Design review of the part built by this model. Coordinates are the model's own, in mm. Coordinates: 2 decimals unless noted, no trailing zeros. Loops run counter-clockwise (first coordinate to the right, second up) from the corner with the lowest first, then second, coordinate; pieces in that order, holes last. Notation, with made-up numbers: M 33,-5 L 80,-5 A9 cw 80,5 Z; hole C 77.25,27.5 d8. An arc over 180 degrees is marked long. Write item = value, one per line. Start each with the question number.
from build123d import *

# Parameters (mm, degrees)
SKETCH1_W           = 38.1
SKETCH1_H           = 28.575
SKETCH1_R           = 3.175
BOSS_EXTRUDE1_DEPTH = 3.175
SKETCH2_R           = 1.8415
CUT_EXTRUDE1_DEPTH  = 25.023234196


with BuildPart() as part:
    # Sketch1 → Boss-Extrude1 (new body)
    with BuildSketch(Plane(origin=(0, 0, 0), x_dir=(1, 0, 0), z_dir=(0, 1, 0))):
        Rectangle(SKETCH1_W, SKETCH1_H)
        with Locations(Location((-10.16, 7.9375, 0), (0, 0, 270))):
            Circle(SKETCH1_R, mode=Mode.SUBTRACT)
    extrude(amount=BOSS_EXTRUDE1_DEPTH)

    # Sketch2 → Cut-Extrude1 (cut, through all)
    with BuildSketch(Plane(origin=(0, 3.175, 0), x_dir=(1, 0, 0), z_dir=(0, 1, 0))):
        with Locations(Location((-14.2875, -9.525, 0), (0, 0, 270))):
            Circle(SKETCH2_R)
        with Locations(Location((14.2875, -9.525, 0), (0, 0, 270))):
            Circle(SKETCH2_R)
        with Locations(Location((14.2875, 9.525, 0), (0, 0, 270))):
            Circle(SKETCH2_R)
    extrude(amount=-CUT_EXTRUDE1_DEPTH, mode=Mode.SUBTRACT)


solid = part.part
Q1. Add section A-A on x = -10.16. State the section outline as (y, z) points (1 decimal), plus the area to 3 significant figures.
Q2. Add section C-C on z = 9.5. State the section outline as (x, y) points (3 decimals), plus the area to 3 significant figures.
Q3. To check wall thickness, follow line 1 (Z direction, x = 14, y = 0.9); line 2 (X direction, y = 2.8, z = 10.5); line 3 (Z direction, x = -12, y = 1.9). State the ranges of each line that lie inside material, in increasing order. Write a range as from..to.
Q4. Mouldability with a two-part tool opening along Z and no side actions: class faces 1 (the face through (12.65, 1.61, -8.68)), 2 (the face through (0, 2, -14.288)), 3 (the face through (-19.05, 2, 0)), 4 (the face through (12.65, 1.61, 10.37)) as released by +Z, released by -Z, zero draft, split by the parting line, or undercut.
Q5. Add section B-B on y = 1.7. Give the number of separate pieces and of enclosed holes in the cut face, plus the area to 3 significant figures.
Values follow:
q1.outline = M 0,-14.3 L 3.2,-14.3 L 3.2,-11.1 L 0,-11.1 Z; M 0,-4.8 L 3.2,-4.8 L 3.2,14.3 L 0,14.3 Z
q1.area = 70.6 mm2
q2.outline = M -19.05,0 L -16.129,0 L -16.129,3.175 L -19.05,3.175 Z; M -12.446,0 L 12.446,0 L 12.446,3.175 L -12.446,3.175 Z; M 16.129,0 L 19.05,0 L 19.05,3.175 L 16.129,3.175 Z
q2.area = 97.6 mm2
q3.line_1 = -14.29..-11.34, -7.71..7.71, 11.34..14.29
q3.line_2 = -19.05..-15.85, -12.73..12.73, 15.85..19.05
q3.line_3 = -14.29..-10.52, -5.35..14.29
q4.face_1 = undercut
q4.face_2 = released by -Z
q4.face_3 = zero draft
q4.face_4 = undercut
q5.separate_pieces = 1
q5.enclosed_holes = 4
q5.area = 1,030 mm2
